Study the drawing (mm; zero at the part's minimum x, y, z) and answer. Coordinates: 2 decimals unless noted, no trailing zeros. Write each loop counter-clockwise with the first axis right and the second up, starting at its lowest first coordinate (ties: lowest second). Pieces come first, ordered by that corner, then holes. Notation, with made-up numbers: (69.25, -23) - (108.25, -23) arc R24 ccw to (108.25, -10) - close; hole circle Ø9 at (89.25, -14). An arc over 180 degrees is marked (long way). One line per item, written item: value.
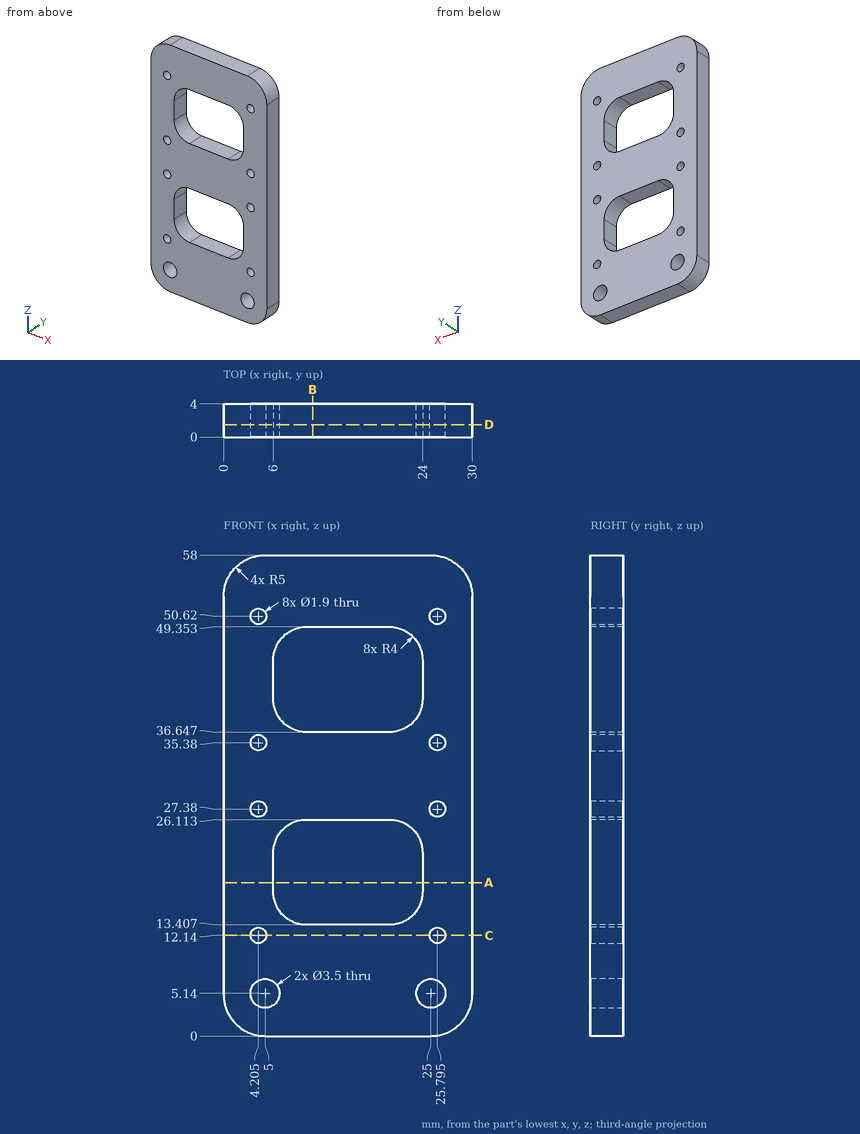
Item 1: Section B-B, the plane x = 10.75 is taken. Determine the outline of the cut face in (y, z), then the cut area to 3 significant figures.
Evaluation:
outline: (0, 0) - (4, 0) - (4, 13.41) - (0, 13.41) - close; (0, 26.11) - (4, 26.11) - (4, 36.65) - (0, 36.65) - close; (0, 49.35) - (4, 49.35) - (4, 58) - (0, 58) - close
area: 130 mm2
Item 2: Consider probe 1 along X at (y, z) = (0.9, 35.38) (3 decimals); probe 2 along Z at (x, y) = (15, 2.5); probe 3 along X at (y, z) = (2.1, 44). Determine where each line is inside the solid, lowest interval first.
Evaluation:
probe 1: x = 0 to 3.255, 5.155 to 24.845, 26.745 to 30
probe 2: z = 0 to 13.41, 26.11 to 36.65, 49.35 to 58
probe 3: x = 0 to 6, 24 to 30
Item 3: Section A-A, the plane z = 18.5 is taken. Determine the outline of the cut face in (x, y), then the cut area to 3 significant figures.
Evaluation:
outline: (0, 0) - (6, 0) - (6, 4) - (0, 4) - close; (24, 0) - (30, 0) - (30, 4) - (24, 4) - close
area: 48.0 mm2
Item 4: Section D-D, the plane y = 1.5 is taken. Give the number of separate pieces and of enclosed holes in the cut face, then the cut area to 3 significant figures.
Evaluation:
separate pieces: 1
enclosed holes: 12
area: 1,250 mm2
Item 5: Section C-C, the plane z = 12.14 is taken. Determine the outline of the cut face in (x, y) (3 decimals).
Evaluation:
outline: (0, 0) - (3.255, 0) - (3.255, 4) - (0, 4) - close; (5.155, 0) - (24.845, 0) - (24.845, 4) - (5.155, 4) - close; (26.745, 0) - (30, 0) - (30, 4) - (26.745, 4) - close
